Part model, mm, in its own coordinate system. A direction names the side the tool comes from. Give positions to 0.01 mm unless a question says otherwise; leave off trailing zeros. Loops run counter-clockwise (first coordinate to the right, second up) from the corner with the lowest first, then second, coordinate; pieces in that order, holes last. Notation, with made-up numbers: (69, -16.75) -> (111, -16.75) arc R32 cw to (111, 17.25) -> close; hole circle Ø3 at (43.25, -16.5). An arc over 180 degrees is marked (long way). Write item = value, one per line.
from build123d import *

# Parameters (mm, degrees)
SKETCH_1_W          = 75.5
SKETCH_1_H          = 51.2
EXTRUDE_1_DEPTH     = 4
HOLE_WIZARD_M3_1_D  = 3.2
FILLET_1_R          = 3
SKETCH_4_W          = 9
SKETCH_4_H          = 11
EXTRUDE_2_DEPTH     = 14
CUT_EXTRUDE_1_DEPTH = 12
SKETCH_6_W          = 25
SKETCH_6_H          = 10
EXTRUDE_3_DEPTH     = 10
SKETCH_7_R          = 1.963016799
CUT_EXTRUDE_2_DEPTH = 1
CHAMFER_1_SIZE      = 2
CHAMFER_1_SIZE2     = 3
SKETCH_8_W          = 8.6
SKETCH_8_H          = 33
EXTRUDE_4_DEPTH     = 10
SKETCH_9_W          = 31
SKETCH_9_H          = 18
EXTRUDE_5_DEPTH     = 14.3
SKETCH_10_W         = 31
SKETCH_10_H         = 14.3
SKETCH_10_R         = 1.542197262
CUT_EXTRUDE_3_DEPTH = 5
SKETCH_11_W         = 16
SKETCH_11_H         = 21
EXTRUDE_6_DEPTH     = 13.4
SKETCH_12_W         = 59.433168898
SKETCH_12_H         = 13.4
CUT_EXTRUDE_4_DEPTH = 0.1
SKETCH_13_W         = 33
SKETCH_13_H         = 10
CUT_EXTRUDE_5_DEPTH = 0.1


with BuildPart() as part:
    # 草图1 → 凸台-拉伸1 (new body)
    with BuildSketch(Plane(origin=(0, 0, 0), x_dir=(1, 0, 0), z_dir=(0, 1, 0))):
        Rectangle(SKETCH_1_W, SKETCH_1_H)
    extrude(amount=EXTRUDE_1_DEPTH)

    # M3 间隙孔1 (through all)
    with Locations(Plane(origin=(0, 4, 0), x_dir=(1, 0, 0), z_dir=(0, 1, 0))):
        with Locations((-35, 23), (35, 23), (-35, -23), (35, -23)):
            Hole(HOLE_WIZARD_M3_1_D / 2)

    # 圆角1
    fillet_1_edges = [part.edges().sort_by_distance(p)[0] for p in [
        (-37.75, 2, -25.6),
        (37.75, 2, -25.6),
        (37.75, 2, 25.6),
        (-37.75, 2, 25.6),
    ]]
    fillet(fillet_1_edges, radius=FILLET_1_R)

    # 草图4 → 凸台-拉伸2 (add)
    with BuildSketch(Plane.XY.offset(25.6)):
        with Locations((23.25, 9.5)):
            Rectangle(SKETCH_4_W, SKETCH_4_H)
    extrude(amount=-EXTRUDE_2_DEPTH)

    # 草图5 → 切除-拉伸1 (cut)
    with BuildSketch(Plane(origin=(0, 0, 11.6), x_dir=(-1, 0, 0), z_dir=(0, 0, -1))):
        with BuildLine():
            Line((-27.75, 10.5), (-28.75, 10.5))
            Line((-28.75, 10.5), (-28.75, 16))
            Line((-28.75, 16), (-17.75, 16))
            Line((-17.75, 16), (-17.75, 10.5))
            Line((-17.75, 10.5), (-18.75, 10.5))
            ThreePointArc((-18.75, 10.5), (-23.25, 15), (-27.75, 10.5))
        make_face()
    extrude(amount=-CUT_EXTRUDE_1_DEPTH, mode=Mode.SUBTRACT)

    # 草图6 → 凸台-拉伸3 (add)
    with BuildSketch(Plane(origin=(0, 4, 0), x_dir=(1, 0, 0), z_dir=(0, 1, 0))):
        with Locations((-1.75, -20.6)):
            Rectangle(SKETCH_6_W, SKETCH_6_H)
    extrude(amount=EXTRUDE_3_DEPTH)

    # 草图7 → 切除-拉伸2 (cut)
    with BuildSketch(Plane(origin=(0, 14, 0), x_dir=(1, 0, 0), z_dir=(0, 1, 0))):
        with Locations(Location((-11.125, -21.230534839, 0), (0, 0, 270))):
            Circle(SKETCH_7_R)
        with Locations(Location((-4.875, -21.230534839, 0), (0, 0, 90))):
            Circle(SKETCH_7_R)
        with Locations(Location((7.625, -21.230534839, 0), (0, 0, 90))):
            Circle(SKETCH_7_R)
        with Locations(Location((1.375, -21.230534839, 0), (0, 0, 270))):
            Circle(SKETCH_7_R)
    extrude(amount=-CUT_EXTRUDE_2_DEPTH, mode=Mode.SUBTRACT)

    # 倒角1
    chamfer_1_edges = [part.edges().sort_by_distance(p)[0] for p in [
        (-1.75, 14, 15.6),
    ]]
    chamfer_1_side = [part.faces().sort_by_distance(p)[0] for p in [
        (-1.75, 9, 15.6),
    ]]
    chamfer(chamfer_1_edges, length=CHAMFER_1_SIZE, length2=CHAMFER_1_SIZE2, reference=chamfer_1_side[0])

    # 草图8 → 凸台-拉伸4 (add)
    with BuildSketch(Plane(origin=(0, 4, 0), x_dir=(1, 0, 0), z_dir=(0, 1, 0))):
        with Locations((33.45, -4.1)):
            Rectangle(SKETCH_8_W, SKETCH_8_H)
    extrude(amount=EXTRUDE_4_DEPTH)

    # 草图9 → 凸台-拉伸5 (add)
    with BuildSketch(Plane(origin=(0, 4, 0), x_dir=(1, 0, 0), z_dir=(0, 1, 0))):
        with Locations((-16.75, 22.6)):
            Rectangle(SKETCH_9_W, SKETCH_9_H)
        with Locations((16.75, 22.6)):
            Rectangle(SKETCH_9_W, SKETCH_9_H)
    extrude(amount=EXTRUDE_5_DEPTH)

    # 草图10 → 切除-拉伸3 (cut)
    # profile 1 of 2: a face of its own
    with BuildSketch(Plane(origin=(0, 0, -31.6), x_dir=(-1, 0, 0), z_dir=(0, 0, -1))):
        with Locations((-16.75, 11.15)):
            Rectangle(SKETCH_10_W, SKETCH_10_H)
        with Locations((-26.769914648, 11.409080509)):
            Circle(SKETCH_10_R, mode=Mode.SUBTRACT)
        with Locations((-6.730085352, 11.409080509)):
            Circle(SKETCH_10_R, mode=Mode.SUBTRACT)
        Polygon((-25.404607637, 8.177619476), (-8.095392363, 8.177619476), (-9.020301502, 15.325154661), (-24.479698498, 15.325154661), align=None, mode=Mode.SUBTRACT)
    # profile 2 of 2: a face of its own
    with BuildSketch(Plane(origin=(0, 0, -31.6), x_dir=(-1, 0, 0), z_dir=(0, 0, -1))):
        with Locations((16.75, 11.15)):
            Rectangle(SKETCH_10_W, SKETCH_10_H)
        with Locations((6.730085352, 11.409080509)):
            Circle(SKETCH_10_R, mode=Mode.SUBTRACT)
        with Locations((26.769914648, 11.409080509)):
            Circle(SKETCH_10_R, mode=Mode.SUBTRACT)
        Polygon((9.020301502, 15.325154661), (8.095392363, 8.177619476), (25.404607637, 8.177619476), (24.479698498, 15.325154661), align=None, mode=Mode.SUBTRACT)
    extrude(amount=-CUT_EXTRUDE_3_DEPTH, mode=Mode.SUBTRACT)

    # 草图11 → 凸台-拉伸6 (add)
    with BuildSketch(Plane(origin=(0, 4, 0), x_dir=(1, 0, 0), z_dir=(0, 1, 0))):
        with Locations((-23.683168898, -15.1)):
            Rectangle(SKETCH_11_W, SKETCH_11_H)
    extrude(amount=EXTRUDE_6_DEPTH)

    # 草图12 → 切除-拉伸4 (cut)
    with BuildSketch(Plane.XY.offset(25.6)):
        with Locations((-1.966584449, 10.7)):
            Rectangle(SKETCH_12_W, SKETCH_12_H)
    extrude(amount=-CUT_EXTRUDE_4_DEPTH, mode=Mode.SUBTRACT)

    # 草图13 → 切除-拉伸5 (cut)
    with BuildSketch(Plane(origin=(37.75, 0, 0), x_dir=(0, 0, -1), z_dir=(1, 0, 0))):
        with Locations((-4.1, 9)):
            Rectangle(SKETCH_13_W, SKETCH_13_H)
    extrude(amount=-CUT_EXTRUDE_5_DEPTH, mode=Mode.SUBTRACT)


solid = part.part
1) Drop flat-ended pins along their axis: P1, Ø8, axis at x = -4.5, y = 15, coming from the +Z side; P2, Ø3, axis at x = -4, z = 20.5, coming from the +Y side; P3, Ø9, axis at x = 1.5, y = 6.5, coming from the -Z side. Give the stop position or say it passes through.
Resolved:
P1 = 25.5
P2 = 14
P3 = -26.6
2) Slice it at B-B, the plane x = 17. List the corners of the cut face in (y, z).
Resolved:
outline = (0, -25.6) -> (4, -25.6) -> (4, -26.6) -> (8.18, -26.6) -> (8.18, -31.6) -> (15.33, -31.6) -> (15.33, -26.6) -> (18.3, -26.6) -> (18.3, -13.6) -> (4, -13.6) -> (4, 25.6) -> (0, 25.6) -> close
3) Pull direction X, two halves, no side cores. Call faces 1 (the face through (-31.683, 11, 15)), 2 (the face through (1.25, 11, -20)), 3 (the face through (-17, 12, -31.6)), 4 (the face through (-25.23, 11.48, -29.14)): pulls with the +X half, pulls with the -X half, needs draft (parallel to the pull), parting line crosses it, or undercut.
Resolved:
face_1 = pulls with the -X half
face_2 = undercut
face_3 = needs draft
face_4 = undercut
4) Slice it at A-A, the plane z = -16. List the corners of the cut face in (x, y).
Resolved:
outline = (-37.75, 0) -> (37.75, 0) -> (37.75, 4) -> (32.25, 4) -> (32.25, 18.3) -> (1.25, 18.3) -> (1.25, 4) -> (-1.25, 4) -> (-1.25, 18.3) -> (-32.25, 18.3) -> (-32.25, 4) -> (-37.75, 4) -> close
5) Slice it at C-C, the plane x = -12. List the corners of the cut face in (y, z), and give its area (3 significant figures).
Resolved:
outline = (0, -25.6) -> (4, -25.6) -> (4, -26.6) -> (8.18, -26.6) -> (8.18, -31.6) -> (15.33, -31.6) -> (15.33, -26.6) -> (18.3, -26.6) -> (18.3, -13.6) -> (4, -13.6) -> (4, 15.6) -> (12, 15.6) -> (14, 18.6) -> (14, 19.47) -> (13, 19.47) -> (13, 22.99) -> (14, 22.99) -> (14, 25.5) -> (4, 25.5) -> (4, 25.6) -> (0, 25.6) -> close
area = 519 mm²
6) Drill centre lines: line 1 along X through (y, z) = (10.25, 19.5); line 2 along Z through (x, y) = (35, 0.8); line 3 along X through (y, z) = (4.75, 21). Where is each one in solid material? Low to high. Write a range as [from, to].
Resolved:
line_1 = [-31.68, -15.68], [-14.25, 10.75], [18.75, 27.75], [29.15, 37.65]
line_2 = [-25.59, -24.6], [-21.4, 21.4], [24.6, 25.59]
line_3 = [-31.68, -15.68], [-14.25, 10.75], [18.75, 27.75]
7) Which spindle directions (+Z, -Z, +X, -X, +Y, -Y) get a long thin tool onto all of the face, cutting with end or side? Do faces 5 (the face through (17, 15.325, -29)), 6 (the face through (10.75, 9, 21)), 7 (the face through (-24, 11, 4.6)), 8 (the face through (-5.19, 11.48, -29.14)). Say none if no direction does.
Resolved:
face_5 = -Z, +X, -X, +Y
face_6 = +Z, +Y
face_7 = -X, +Y
face_8 = -Z
8) Slice it at D-D, the plane z = 17. List the corners of the cut face in (x, y), and give its area (3 significant figures).
Resolved:
outline = (-37.75, 0) -> (37.75, 0) -> (37.75, 4) -> (37.65, 4) -> (37.65, 14) -> (29.15, 14) -> (29.15, 4) -> (27.75, 4) -> (27.75, 10.5) arc R4.5 ccw to (18.75, 10.5) -> (18.75, 4) -> (10.75, 4) -> (10.75, 12.93) -> (-14.25, 12.93) -> (-14.25, 4) -> (-15.68, 4) -> (-15.68, 17.4) -> (-31.68, 17.4) -> (-31.68, 4) -> (-37.75, 4) -> close
area = 915 mm²
